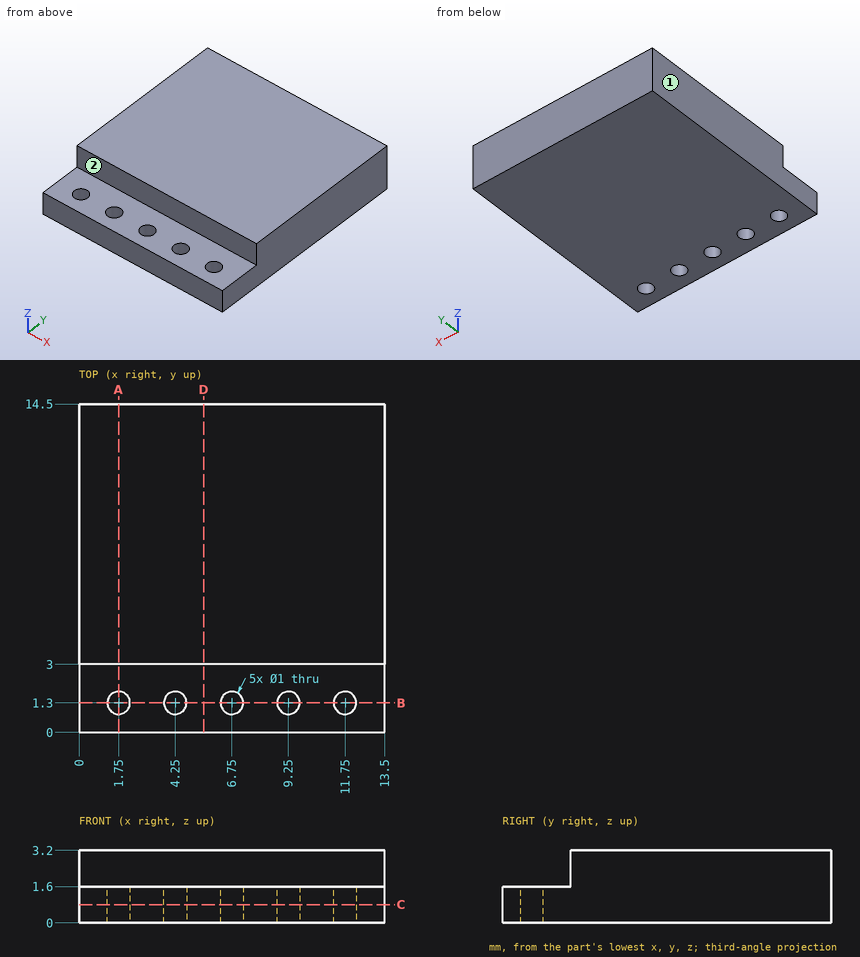
The figure shows three views and two pictorial views of one solid part (mm, origin at its lowest corner). Answer the questions. A direction names the side the tool comes from. Round coordinates to 2 decimals unless told otherwise and drop trailing zeros. Write each loop counter-clockwise with the first axis right and the second up, starting at its lowest first coordinate (ties: lowest second). Pieces come first, ordered by that corner, then holes. Notation, with made-up numbers: (62.5, 83.25) -> (85.5, 83.25) arc R27 cw to (85.5, 110.25) -> close; hole circle Ø4 at (62.25, 18.5). An arc over 180 degrees is marked (long way). Answer as a JSON object with one key per item and string values. Group by question number.
Q1. Section A-A (x = 1.75) is taken. Write down the section's boundary in (y, z).
Q2. Section B-B (y = 1.3) is taken. Write down the section's boundary in (x, z), plus the area to 3 significant figures.
Q3. Each of these flat-tipped pins is pushed along its axis until it touches: pin 1 Ø8 at (x, y) = (7.5, 11.5) entering from -Z; pin 2 Ø2.5 at (x, y) = (9.5, 1.5) entering from +Z. Where does it stop, or does it pass through?
Q4. Which of the six approach directions +Z, -Z, +X, -X, +Y, -Y give full straight-line access (tool end or side, diameter ignored) to the marked faces 1 and 2?
Q5. Section C-C (z = 0.8) is taken. Write down the section's boundary in (x, y).
Q6. Straight lines are drawn through the part: line 1 along Y through (x, z) = (6.75, 0.8); line 2 along Y through (x, z) = (4, 2.35); line 3 along Z through (x, y) = (9, 2.25). For each, find the intervals that lie inside material, in ascending order.
Q7. Section D-D (x = 5.5) is taken. Write down the section's boundary in (y, z), plus the area to 3 significant figures.
Check values:
{
 "1": {"outline": "(0, 0) -> (0.8, 0) -> (0.8, 1.6) -> (0, 1.6) -> close; (1.8, 0) -> (14.5, 0) -> (14.5, 3.2) -> (3, 3.2) -> (3, 1.6) -> (1.8, 1.6) -> close"},
 "2": {"outline": "(0, 0) -> (1.25, 0) -> (1.25, 1.6) -> (0, 1.6) -> close; (2.25, 0) -> (3.75, 0) -> (3.75, 1.6) -> (2.25, 1.6) -> close; (4.75, 0) -> (6.25, 0) -> (6.25, 1.6) -> (4.75, 1.6) -> close; (7.25, 0) -> (8.75, 0) -> (8.75, 1.6) -> (7.25, 1.6) -> close; (9.75, 0) -> (11.25, 0) -> (11.25, 1.6) -> (9.75, 1.6) -> close; (12.25, 0) -> (13.5, 0) -> (13.5, 1.6) -> (12.25, 1.6) -> close", "area": "13.6 mm^2"},
 "3": {"pin 1": "z = 0", "pin 2": "z = 1.6"},
 "4": {"face 1": "+Z, -Z, -X, +Y, -Y", "face 2": "+Z, +X, -X, -Y"},
 "5": {"outline": "(0, 0) -> (13.5, 0) -> (13.5, 14.5) -> (0, 14.5) -> close; hole circle Ø1 at (1.75, 1.3); hole circle Ø1 at (4.25, 1.3); hole circle Ø1 at (6.75, 1.3); hole circle Ø1 at (9.25, 1.3); hole circle Ø1 at (11.75, 1.3)"},
 "6": {"line 1": "0 to 0.8, 1.8 to 14.5", "line 2": "3 to 14.5", "line 3": "0 to 1.6"},
 "7": {"outline": "(0, 0) -> (14.5, 0) -> (14.5, 3.2) -> (3, 3.2) -> (3, 1.6) -> (0, 1.6) -> close", "area": "41.6 mm^2"}
}
